Geometry check sheet. Reference: the model listing, model coordinates, mm. A direction names the side the tool comes from. Coordinates: 2 decimals unless noted, no trailing zeros. Write each loop counter-clockwise with the first axis right and the second up, starting at its lowest first coordinate (ties: lowest second). Pieces come first, ordered by that corner, then holes. Notation, with made-up numbers: (-4, 89) -> (39, 89) arc R16 ccw to (39, 94) -> close; hole circle Ø8 at (21, -8). An arc over 180 degrees is marked (long way). Answer as CSV lines item,"result".
```python
from build123d import *

# Parameters (mm, degrees)
EXTRUDE1_START     = -9.35
SKETCH1_R          = 2
EXTRUDE1_DEPTH     = 20
EXTRUDE2_START     = -10.65
SKETCH6_R          = 3.5
EXTRUDE2_DEPTH     = 1.3
CUT_EXTRUDE1_DEPTH = 0.975
SKETCH8_R          = 1.443375673
CUT_EXTRUDE2_DEPTH = 0.975
CUT_EXTRUDE2_TAPER = 45
CHAMFER1_SIZE      = 0.1625
CHAMFER2_SIZE      = 0.525


with BuildPart() as part:
    # Sketch1 → Extrude1 (new body)
    with BuildSketch(Plane.XY.offset(EXTRUDE1_START)):
        Circle(SKETCH1_R)
    extrude(amount=EXTRUDE1_DEPTH)

    # Sketch6 → Extrude2 (add)
    with BuildSketch(Plane.XY.offset(EXTRUDE2_START)):
        Circle(SKETCH6_R)
    extrude(amount=EXTRUDE2_DEPTH)

    # Sketch7 → Cut-Extrude1 (cut)
    with BuildSketch(Plane.XY.offset(-10.65)):
        Polygon((0, 1.443375673), (-1.25, 0.721687836), (-1.25, -0.721687836), (0, -1.443375673), (1.25, -0.721687836), (1.25, 0.721687836), align=None)
    extrude(amount=CUT_EXTRUDE1_DEPTH, mode=Mode.SUBTRACT)

    # Sketch8 → Cut-Extrude2 (cut)
    with BuildSketch(Plane.XY.offset(-10.65)):
        Circle(SKETCH8_R)
    extrude(amount=CUT_EXTRUDE2_DEPTH, taper=CUT_EXTRUDE2_TAPER, mode=Mode.SUBTRACT)

    # Chamfer1
    chamfer1_edges = [part.edges().sort_by_distance(p)[0] for p in [
        (-3.5, 0, -9.35),
        (-3.5, 0, -10.65),
    ]]
    chamfer(chamfer1_edges, length=CHAMFER1_SIZE)

    # Chamfer2
    chamfer2_edges = [part.edges().sort_by_distance(p)[0] for p in [
        (-2, 0, 10.65),
    ]]
    chamfer(chamfer2_edges, length=CHAMFER2_SIZE)


solid = part.part
```
Item 1: Release check for a two-part mould opening along Y. For faces 4 (the flat face through (0.69, -1.44, -10.65)), 5 (the cylindrical face through (3.233, -1.341, -10.007)), 6 (the flat face through (0.63, 1.08, -10.06)), 7 (the flat face through (-0.63, -1.08, -10.06)) record: +Y half, -Y half, draft (parallel to the pull), parting line (faces both ways), or undercut.
Responses:
face 4,"draft"
face 5,"parting line"
face 6,"undercut"
face 7,"undercut"
Item 2: Cross-section at B-B, the plane z = -9. Record the cut outline in (x, y), plus the area to 3 significant figures.
Responses:
outline,"circle Ø4 at (0, 0)"
area,"12.6 mm2"
Item 3: Thickness scan on probe 1 along Z at (x, y) = (2, -1.25); probe 2 along Y at (x, z) = (0, 2.5); probe 3 along X at (y, z) = (-0.25, -4.25). Record the ranges inside material, lowest first.
Responses:
probe 1,"z = -10.65 to -9.35"
probe 2,"y = -2 to 2"
probe 3,"x = -1.98 to 1.98"
Item 4: Depth check by flat-ended pin: pin 1 Ø4 at (y, z) = (2, 7) entering from -X; pin 2 Ø2 at (x, z) = (0, 4.5) entering from -Y. Enter the tip coordinate at first touch or a pass-through.
Responses:
pin 1,"stops at x = -2"
pin 2,"stops at y = -2"
Item 5: Set-up check for faces 1 (the flat face through (0, 0, 10.65)), 2 (the flat face through (0, -2.2, -9.35)), 3 (the flat face through (0.616, -1.088, -10.061)): record each of +Z, -Z, +X, -X, +Y, -Y from which the full face is reachable in a straight line by a thin tool's end or side.
Responses:
face 1,"+Z, +X, -X, +Y, -Y"
face 2,"+Z"
face 3,"-Z"
